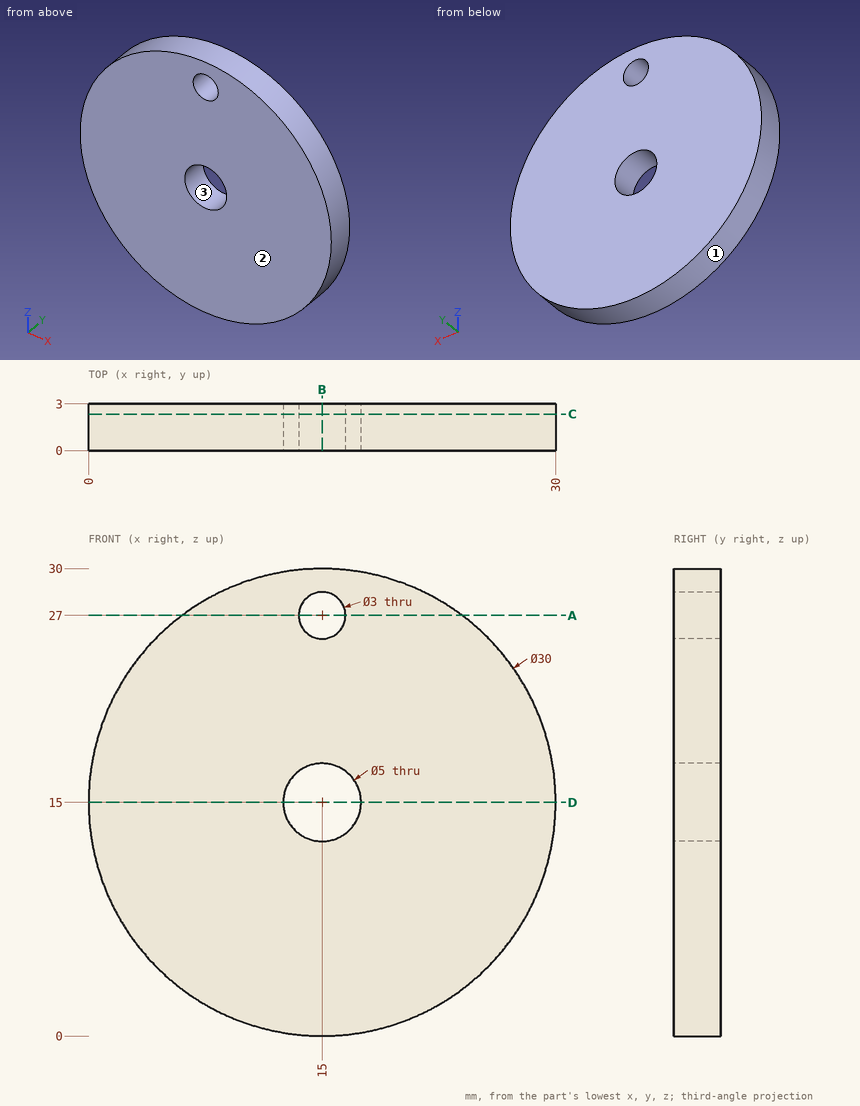
Answer from the drawing. Dimensions are ordinates in mm from the lowest x, y and z of the part. Give positions to 0.01 mm unless a question says otherwise; leave off trailing zeros. Loops run counter-clockwise (first coordinate to the right, second up) from the corner with the lowest first, then second, coordinate; pieces in that order, holes last.
Item 1: Determine the mould class of the marked faces 1, 2 and 3 for opening direction Z: +Z half, -Z half, draft (parallel to the pull), parting line (faces both ways), or undercut.
Derived:
face 1: parting line
face 2: draft
face 3: undercut
Item 2: A cutting plane is placed at C-C (y = 2.35). Give the vertices of the cut face in (x, z), then the cut area to 3 significant figures.
Derived:
outline: circle Ø30 at (15, 15); hole circle Ø5 at (15, 15); hole circle Ø3 at (15, 27)
area: 680 mm2
Item 3: A cutting plane is placed at D-D (z = 15). Give the vertices of the cut face in (x, y), then the cut area to 3 significant figures.
Derived:
outline: (0, 0) - (12.5, 0) - (12.5, 3) - (0, 3) - close; (17.5, 0) - (30, 0) - (30, 3) - (17.5, 3) - close
area: 75.0 mm2
Item 4: Find the intervals of material crossed by line 1 along Z through (x, y) = (15, 1.6); line 2 along X through (y, z) = (2.45, 17); line 3 along X through (y, z) = (2.55, 23.75), in increasing order.
Derived:
line 1: z = 0 to 12.5, 17.5 to 25.5, 28.5 to 30
line 2: x = 0.13 to 13.5, 16.5 to 29.87
line 3: x = 2.82 to 27.18
Item 5: A cutting plane is placed at A-A (z = 27). Give the vertices of the cut face in (x, y).
Derived:
outline: (6, 0) - (13.5, 0) - (13.5, 3) - (6, 3) - close; (16.5, 0) - (24, 0) - (24, 3) - (16.5, 3) - close
Item 6: A cutting plane is placed at B-B (x = 15). Give the vertices of the cut face in (y, z).
Derived:
outline: (0, 0) - (3, 0) - (3, 12.5) - (0, 12.5) - close; (0, 17.5) - (3, 17.5) - (3, 25.5) - (0, 25.5) - close; (0, 28.5) - (3, 28.5) - (3, 30) - (0, 30) - close
